Here's how the part is built. I have some questions about the finished solid (model axes, mm). Give positions to 0.01 mm unless a question says otherwise; leave off trailing zeros. Loops run counter-clockwise (first coordinate to the right, second up) from the corner with the lowest first, then second, coordinate; pieces in that order, holes last. Notation, with made-up numbers: (-13.5, 27) - (14.5, 27) arc R23 cw to (14.5, 64) - close; hole circle Ø6 at (62, -5). An arc over 180 degrees is marked (long way). Use a Markdown table: item, result.
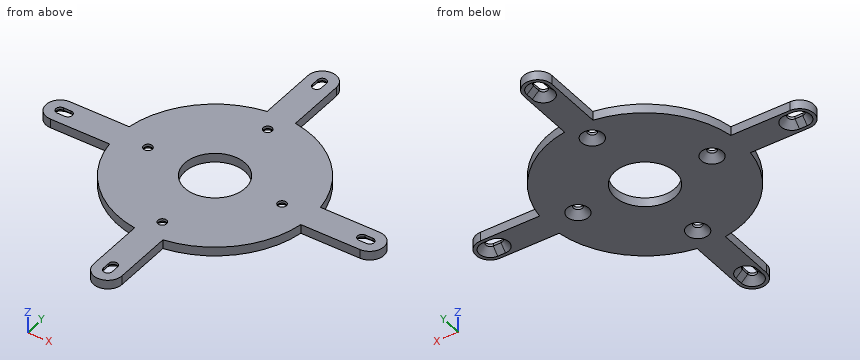
from build123d import *

# Parameters (mm, degrees)
SKETCH1_R           = 37.5
BOSS_EXTRUDE1_DEPTH = 3.5
SKETCH1_3_R         = 1.7
CUT_EXTRUDE1_DEPTH  = 13
CHAMFER1_SIZE       = 2.5
SKETCH2_R           = 11.692051929
CUT_EXTRUDE2_DEPTH  = 10


with BuildPart() as part:
    # Sketch1 → Boss-Extrude1 (new body)
    # profile 1 of 3: a face of its own
    with BuildSketch(Plane.XY):
        Circle(SKETCH1_R)
    # profile 2 of 3: a face of its own
    with BuildSketch(Plane.XY):
        with BuildLine():
            Line((60, -5.5), (-60, -5.5))
            ThreePointArc((-60, -5.5), (-65.5, 0), (-60, 5.5))
            Line((-60, 5.5), (60, 5.5))
            ThreePointArc((60, 5.5), (65.5, 0), (60, -5.5))
        make_face()
        with BuildLine():
            Line((-60, 1.7), (-57, 1.7))
            ThreePointArc((-57, 1.7), (-55.3, 0), (-57, -1.7))
            Line((-57, -1.7), (-60, -1.7))
            ThreePointArc((-60, -1.7), (-61.7, 0), (-60, 1.7))
        make_face(mode=Mode.SUBTRACT)
        with BuildLine():
            Line((60, -1.7), (57, -1.7))
            ThreePointArc((57, -1.7), (55.3, 0), (57, 1.7))
            Line((57, 1.7), (60, 1.7))
            ThreePointArc((60, 1.7), (61.7, 0), (60, -1.7))
        make_face(mode=Mode.SUBTRACT)
    # profile 3 of 3: a face of its own
    with BuildSketch(Plane.XY):
        with BuildLine():
            Line((-5.5, -60), (-5.5, 60))
            ThreePointArc((-5.5, 60), (0, 65.5), (5.5, 60))
            Line((5.5, 60), (5.5, -60))
            ThreePointArc((5.5, -60), (0, -65.5), (-5.5, -60))
        make_face()
        with BuildLine():
            Line((-1.7, -60), (-1.7, -57))
            ThreePointArc((-1.7, -57), (0, -55.3), (1.7, -57))
            Line((1.7, -57), (1.7, -60))
            ThreePointArc((1.7, -60), (0, -61.7), (-1.7, -60))
        make_face(mode=Mode.SUBTRACT)
        with BuildLine():
            Line((1.7, 60), (1.7, 57))
            ThreePointArc((1.7, 57), (0, 55.3), (-1.7, 57))
            Line((-1.7, 57), (-1.7, 60))
            ThreePointArc((-1.7, 60), (0, 61.7), (1.7, 60))
        make_face(mode=Mode.SUBTRACT)
    extrude(amount=BOSS_EXTRUDE1_DEPTH)

    # Sketch1_3 → Cut-Extrude1 (cut)
    with BuildSketch(Plane.XY):
        with Locations(Location((0, 29.5, 0), (0, 0, 180))):
            Circle(SKETCH1_3_R)
        with Locations(Location((26, 0, 0), (0, 0, 180))):
            Circle(SKETCH1_3_R)
        with Locations(Location((-26, 0, 0), (0, 0, 180))):
            Circle(SKETCH1_3_R)
        with Locations(Location((0, -29.5, 0), (0, 0, 180))):
            Circle(SKETCH1_3_R)
    extrude(amount=CUT_EXTRUDE1_DEPTH, mode=Mode.SUBTRACT)

    # Chamfer1
    chamfer1_edges = [part.edges().sort_by_distance(p)[0] for p in [
        (-24.3, 0, 0),
        (1.7, 29.5, 0),
        (1.7, -29.5, 0),
        (27.7, 0, 0),
        (-1.7, -58.5, 0),
        (0, -61.7, 0),
        (1.7, -58.5, 0),
        (0, -55.3, 0),
        (58.5, -1.7, 0),
        (61.7, 0, 0),
        (58.5, 1.7, 0),
        (55.3, 0, 0),
        (1.7, 58.5, 0),
        (0, 61.7, 0),
        (-1.7, 58.5, 0),
        (0, 55.3, 0),
        (-58.5, 1.7, 0),
        (-61.7, 0, 0),
        (-58.5, -1.7, 0),
        (-55.3, 0, 0),
    ]]
    chamfer(chamfer1_edges, length=CHAMFER1_SIZE)

    # Sketch2 → Cut-Extrude2 (cut)
    with BuildSketch(Plane(origin=(0, 0, 0), x_dir=(-1, 0, 0), z_dir=(0, 0, -1))):
        Circle(SKETCH2_R)
    extrude(amount=-CUT_EXTRUDE2_DEPTH, mode=Mode.SUBTRACT)


solid = part.part
(1) Will these pins go through, and if not, where does the flat tip stop? pin 1 (1.8 mm diameter, centred on x = 54, z = 2, fed in from -Y); pin 2 (1.5 mm diameter, centred on y = -15, z = 2.5, fed in from +X); pin 3 (4 mm diameter, centred on x = 0, y = -29.5, fed in from -Z).
A:
| item | result |
|---|---|
| pin 1 | y = -5.5 |
| pin 2 | x = 34.69 |
| pin 3 | z = 2.2 |
(2) If I drill on line 1 (Y direction, x = 0, z = 2.3); line 2 (Y direction, x = 0, z = 1.45); line 3 (Y direction, x = -51, z = 2), over which ranges is the centre line in solid material (lowest first)?
A:
| item | result |
|---|---|
| line 1 | -65.5 to -61.9, -55.1 to -31.4, -27.6 to -11.69, 11.69 to 27.6, 31.4 to 55.1, 61.9 to 65.5 |
| line 2 | -65.5 to -62.75, -54.25 to -32.25, -26.75 to -11.69, 11.69 to 26.75, 32.25 to 54.25, 62.75 to 65.5 |
| line 3 | -5.5 to 5.5 |
(3) Suppose I cut it at C-C on y = 8.5. Write out the boundary of the cut face in (x, z), plus the area to 3 significant figures.
A:
| item | result |
|---|---|
| outline | (-36.52, 0) - (-8.03, 0) - (-8.03, 3.5) - (-36.52, 3.5) - close; (8.03, 0) - (36.52, 0) - (36.52, 3.5) - (8.03, 3.5) - close |
| area | 199 mm2 |
(4) Suppose I cut it at D-D on x = 7.5. Write out the boundary of the cut face in (y, z).
A:
| item | result |
|---|---|
| outline | (-36.74, 0) - (-8.97, 0) - (-8.97, 3.5) - (-36.74, 3.5) - close; (8.97, 0) - (36.74, 0) - (36.74, 3.5) - (8.97, 3.5) - close |
(5) Suppose I cut it at B-B on z = 1.6. Count the separate pieces of the cut face and the enclosed holes in it, plus the area to 3 significant figures.
A:
| item | result |
|---|---|
| separate pieces | 1 |
| enclosed holes | 9 |
| area | 4,940 mm2 |
(6) Suppose I cut it at A-A on x = -26. Write out the boundary of the cut face in (y, z), plus the area to 3 significant figures.
A:
| item | result |
|---|---|
| outline | (-27.02, 0) - (-4.2, 0) - (-1.7, 2.5) - (-1.7, 3.5) - (-27.02, 3.5) - close; (1.7, 2.5) - (4.2, 0) - (27.02, 0) - (27.02, 3.5) - (1.7, 3.5) - close |
| area | 171 mm2 |
